```python
from build123d import *

# Parameters (mm, degrees)
F1_DEPTH = 0.5
F2_W     = 80
F2_H     = 3
F3_DEPTH = 6
F4_W     = 2
F4_H     = 7
F5_DEPTH = 80
F6_SIZE  = 2


with BuildPart() as f1:
    # F0 (on Right) → F1 (new body)
    with BuildSketch(Plane.YZ):
        with BuildLine():
            ThreePointArc((-50, -10), (-48.535534, -13.535534), (-45, -15))
            Line((-45, -15), (45, -15))
            ThreePointArc((45, -15), (48.535534, -13.535534), (50, -10))
            Line((50, -10), (50, 10))
            ThreePointArc((50, 10), (48.535534, 13.535534), (45, 15))
            Line((45, 15), (-45, 15))
            ThreePointArc((-45, 15), (-48.535534, 13.535534), (-50, 10))
            Line((-50, 10), (-50, -10))
        make_face()
    extrude(amount=F1_DEPTH)

    # F2 (on face) → F3 (join)
    with BuildSketch(Plane(origin=(0, 0, 0), x_dir=(0, -1, 0), z_dir=(-1, 0, 0))):
        with Locations((0, 11.5)):
            Rectangle(F2_W, F2_H)
        with Locations((0, -11.5)):
            Rectangle(F2_W, F2_H)
    extrude(amount=F3_DEPTH)

    # F4 (on face) → F5 (cut)
    with BuildSketch(Plane(origin=(0, 0, -13), x_dir=(1, 0, 0), z_dir=(0, 0, -1))):
        with Locations((-2, -26.5)):
            Rectangle(F4_W, F4_H)
        with Locations((-2, 26.5)):
            Rectangle(F4_W, F4_H)
    extrude(amount=-F5_DEPTH, mode=Mode.SUBTRACT)

    # F6
    f6_edges = [f1.edges().sort_by_distance(p)[0] for p in [
        (-6, 0, -10),
        (-6, 0, 10),
    ]]
    chamfer(f6_edges, length=F6_SIZE)


solid = f1.part
```
Build history of the part. All positions in model axes, mm. A direction names the side the tool comes from. Round coordinates to 2 decimals unless told otherwise and drop trailing zeros. Loops run counter-clockwise (first coordinate to the right, second up) from the corner with the lowest first, then second, coordinate; pieces in that order, holes last. Notation, with made-up numbers: M 17.25,68 L 61.25,68 A22 cw 61.25,81 Z; hole C 80.5,88 d4. An arc over 180 degrees is marked long. Answer as CSV lines item,"result".
1. Cut at C-C on z = 3. Write the cut outline in (x, y), then the cut area to 3 significant figures.
Resolved:
outline,"M 0,-50 L 0.5,-50 L 0.5,50 L 0,50 Z"
area,"50.0 mm²"
2. Cut at A-A on y = 24. Write the cut outline in (x, z), then the cut area to 3 significant figures.
Resolved:
outline,"M -6,-13 L -3,-13 L -3,-10 L -4,-10 L -6,-12 Z; M -6,12 L -4,10 L -3,10 L -3,13 L -6,13 Z; M -1,-13 L 0,-13 L 0,-15 L 0.5,-15 L 0.5,15 L 0,15 L 0,13 L -1,13 L -1,10 L 0,10 L 0,-10 L -1,-10 Z"
area,"35.0 mm²"
3. 3-axis set-ups, long thin cutter, end or side, ignore diameter. For faces 5 (the flat face through (-3, 1, -13)), 6 (the flat face through (-3, 40, 11)), 7 (the flat face through (-2, 1, 10)), 8 (the flat face through (-2, -30, -12)): which of +Z, -Z, +X, -X, +Y, -Y reach the whole face in a straight line?
Resolved:
face 5,"-Z, -X, +Y, -Y"
face 6,"+Z, -Z, -X, +Y"
face 7,"-X, +Y, -Y"
face 8,"+Z, -Z"
4. Two-plate mould, pull along Z, no slides. Class faces 1 (the flat face through (-3, 1, 13)), 2 (the flat face through (-2, 1, -10)), 3 (the flat face through (-1, 27, -12)), 4 (the flat face through (0, -1, 0)): released by +Z, released by -Z, zero draft, split by the parting line, or undercut.
Resolved:
face 1,"released by +Z"
face 2,"undercut"
face 3,"zero draft"
face 4,"undercut"
5. Flat gauge pins, fed straight in: P1, Ø1.5, axis at x = -2, z = 7.5, coming from the +Y side; P2, Ø2.5, axis at x = -4, z = 11, coming from the +Y side; P3, Ø1.2, axis at x = -1, y = -2.5, coming from the -Z side; P4, Ø2, axis at x = -2, z = -12, coming from the -Y side. Where does each tip first touch, or does it go through?
Resolved:
P1,"passes through"
P2,"stops at y = 40"
P3,"stops at z = -13"
P4,"stops at y = -40"
6. Cut at B-B on y = 1. Write the cut outline in (x, z), then the cut area to 3 significant figures.
Resolved:
outline,"M -6,-13 L 0,-13 L 0,-15 L 0.5,-15 L 0.5,15 L 0,15 L 0,13 L -6,13 L -6,12 L -4,10 L 0,10 L 0,-10 L -4,-10 L -6,-12 Z"
area,"47.0 mm²"
7. Wall check: probe 1 along Y at (x, z) = (-1.75, -11); probe 2 along Z at (x, y) = (-2.75, 33.5); probe 3 along X at (y, z) = (40, -9). Give the ranges that are in metal, low to high. Write a range as [from, to].
Resolved:
probe 1,"y = [-40, -30], [-23, 23], [30, 40]"
probe 2,"z = [-13, -10], [10, 13]"
probe 3,"x = [0, 0.5]"
